Model file for the job. Use its own axes, mm. Face numbers are marked on the shaded views. A direction names the side the tool comes from. Coordinates: 2 decimals unless noted, no trailing zeros. Write each loop counter-clockwise with the first axis right and the second up, starting at its lowest first coordinate (ties: lowest second). Pieces come first, ordered by that corner, then holes. Notation, with made-up numbers: M -1,-6 L 48,-6 A25 ccw 48,29 Z; hole C 77.25,31 d2. An arc over 180 degrees is marked long. Put each result on its own line as item: value. Start each with the question number.
Q1. Drop a flat-ended pin along its axis: pin 1 (1.8 mm diameter, centred on x = 17.35, y = 6.5, fed in from +Z). Give the stop position or say it passes through.
Q2. Drill centre lines: line 1 along Y through (x, z) = (17.35, 1.1); line 2 along Y through (x, z) = (27, 2.35); line 3 along Y through (x, z) = (8.5, 2.2). Where is each one in solid material? Low to high.
Q3. Which spindle directions (+Z, -Z, +X, -X, +Y, -Y) get a long thin tool onto all of the face, cutting with end or side? Do the marked faces 4 and 5. Say none if no direction does.
Q4. Cut at D-D (x = 27). Write the cut outline in (y, z).
Q5. Cut at A-A (y = 6.5). Write the cut outline in (x, z).
Q6. Cut at C-C (z = 0.45). Give the number of separate pieces and of enclosed holes in the cut face, then the cut area to 3 significant figures.
Q7. Cut at B-B (x = 17.35). Write the cut outline in (y, z), then the cut area to 3 significant figures.
Q8. Pull direction Y, two halves, no side cores. Call the marked faces 1, 2 and 3: pulls with the +Y half, pulls with the -Y half, needs draft (parallel to the pull), parting line crosses it, or undercut.
```python
from build123d import *

# Parameters (mm, degrees)
ESQUISSE1_W             = 32
ESQUISSE1_H             = 13
ESQUISSE1_R             = 2.3
ESQUISSE1_R_2           = 1
BOSS_EXTRU_1_DEPTH      = 3
ENL_V_MAT_EXTRU_1_DEPTH = 1.5


with BuildPart() as part:
    # Esquisse1 → Boss.-Extru.1 (new body)
    with BuildSketch(Plane.XY):
        with Locations((16, 6.5)):
            Rectangle(ESQUISSE1_W, ESQUISSE1_H)
        with Locations((5, 6.5)):
            Circle(ESQUISSE1_R, mode=Mode.SUBTRACT)
        with Locations((27, 6.5)):
            Circle(ESQUISSE1_R, mode=Mode.SUBTRACT)
        with Locations((14.65, 9.2)):
            Circle(ESQUISSE1_R_2, mode=Mode.SUBTRACT)
        with Locations((17.35, 9.2)):
            Circle(ESQUISSE1_R_2, mode=Mode.SUBTRACT)
        with Locations((17.35, 6.5)):
            Circle(ESQUISSE1_R_2, mode=Mode.SUBTRACT)
        with Locations((14.65, 3.8)):
            Circle(ESQUISSE1_R_2, mode=Mode.SUBTRACT)
        with Locations((14.65, 6.5)):
            Circle(ESQUISSE1_R_2, mode=Mode.SUBTRACT)
        with Locations((17.35, 3.8)):
            Circle(ESQUISSE1_R_2, mode=Mode.SUBTRACT)
    extrude(amount=BOSS_EXTRU_1_DEPTH)

    # Esquisse2 → Enlèv. mat.-Extru.1 (cut)
    with BuildSketch(Plane.XY.offset(3)):
        with BuildLine():
            Line((1.5, 11.5), (13.670204103, 11.5))
            ThreePointArc((13.670204103, 11.5), (12.260789898, 9.935985793), (12.545837459, 7.85))
            ThreePointArc((12.545837459, 7.85), (12.15, 6.5), (12.545837459, 5.15))
            ThreePointArc((12.545837459, 5.15), (12.260789898, 3.064014207), (13.670204103, 1.5))
            Line((13.670204103, 1.5), (1.5, 1.5))
            Line((1.5, 1.5), (1.5, 5.020135141))
            ThreePointArc((1.5, 5.020135141), (8.8, 6.5), (1.5, 7.979864859))
            Line((1.5, 7.979864859), (1.5, 11.5))
        make_face()
        with BuildLine():
            Line((30.5, 1.5), (18.329795897, 1.5))
            ThreePointArc((18.329795897, 1.5), (19.739210102, 3.064014207), (19.454162541, 5.15))
            ThreePointArc((19.454162541, 5.15), (19.85, 6.5), (19.454162541, 7.85))
            ThreePointArc((19.454162541, 7.85), (19.739210102, 9.935985793), (18.329795897, 11.5))
            Line((18.329795897, 11.5), (30.5, 11.5))
            Line((30.5, 11.5), (30.5, 7.979864859))
            ThreePointArc((30.5, 7.979864859), (23.2, 6.5), (30.5, 5.020135141))
            Line((30.5, 5.020135141), (30.5, 1.5))
        make_face()
    extrude(amount=-ENL_V_MAT_EXTRU_1_DEPTH, mode=Mode.SUBTRACT)


solid = part.part
```
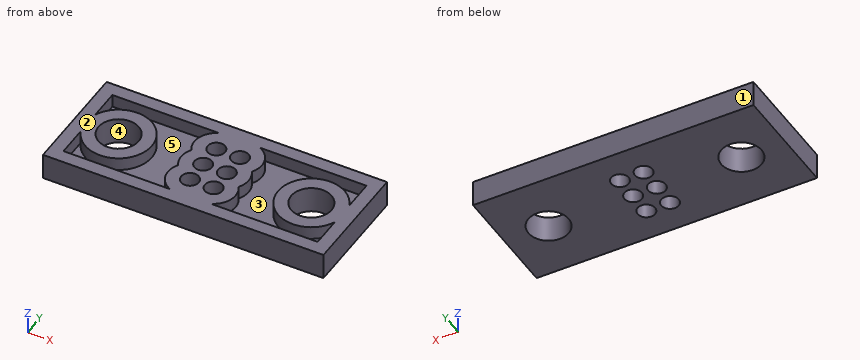
Computed values:
1. pin 1: through
2. line 1: 0 to 2.8, 4.8 to 5.5, 7.5 to 8.2, 10.2 to 13
2. line 2: 0 to 1.5, 2.7 to 4.2, 8.8 to 10.3, 11.5 to 13
2. line 3: 0 to 1.5, 5.02 to 7.98, 11.5 to 13
3. face 4: +Z, -Z
3. face 5: +Z
4. outline: M 0,0 L 4.2,0 L 4.2,3 L 2.7,3 L 2.7,1.5 L 1.5,1.5 L 1.5,3 L 0,3 Z; M 8.8,0 L 13,0 L 13,3 L 11.5,3 L 11.5,1.5 L 10.3,1.5 L 10.3,3 L 8.8,3 Z
5. outline: M 0,0 L 2.7,0 L 2.7,3 L 0,3 Z; M 7.3,0 L 13.65,0 L 13.65,3 L 12.15,3 L 12.15,1.5 L 8.8,1.5 L 8.8,3 L 7.3,3 Z; M 15.65,0 L 16.35,0 L 16.35,3 L 15.65,3 Z; M 18.35,0 L 24.7,0 L 24.7,3 L 23.2,3 L 23.2,1.5 L 19.85,1.5 L 19.85,3 L 18.35,3 Z; M 29.3,0 L 32,0 L 32,3 L 29.3,3 Z
6. separate pieces: 1
6. enclosed holes: 8
6. area: 364 mm2
7. outline: M 0,0 L 2.8,0 L 2.8,3 L 0,3 Z; M 4.8,0 L 5.5,0 L 5.5,3 L 4.8,3 Z; M 7.5,0 L 8.2,0 L 8.2,3 L 7.5,3 Z; M 10.2,0 L 13,0 L 13,3 L 10.2,3 Z
7. area: 21.0 mm2
8. face 1: pulls with the +Y half
8. face 2: needs draft
8. face 3: undercut
